Design review of the part built by this model. Coordinates are the model's own, in mm. Coordinates: 2 decimals unless noted, no trailing zeros. Write each loop counter-clockwise with the first axis right and the second up, starting at its lowest first coordinate (ties: lowest second). Pieces come first, ordered by that corner, then holes.
Q1. For probe 1 along Z at (x, y) = (-0.5, -9.25); probe 2 along Z at (x, y) = (0, -3.5); probe 3 along Y at (x, z) = (-6, 33.5), list the stretches that pass through material, from the lowest coordinate up.
Q2. Take a section at D-D (y = 1.25). Give the boundary of the cut face in (x, z), and give its area (3 significant figures).
Q3. Insertion check: pin 1 (5 mm diameter, centred on x = -1.5, y = -7, fed in from +Z); pin 2 (0.5 mm diameter, centred on y = -8.5, z = 34, fed in from -X); pin 3 (6 mm diameter, centred on x = 2.5, z = -28.5, fed in from -Y). Each pin has a flat end and moves straight along its axis. Give the tip position at first contact, or say it passes through.
Q4. Take a section at B-B (y = -5.25). Give the boundary of the cut face in (x, z), and give its area (3 significant figures).
Autodesk Fusion 360 part; units mm, degrees
sketch "Sketch1" plane through (0, 0, 0) normal (0, 1, 0) x (1, 0, 0)
  line L0 (10, 40) -> (-10, 40)
  line L1 (-10, 40) -> (-10, -40)
  line L2 (-10, -40) -> (10, -40)
  line L3 (10, -40) -> (10, 40)
  line L4 (10, 40) -> (-10, -40) construction
  line L5 (-10, 40) -> (10, -40) construction
  dimension "d1" = 20
  dimension "d2" = 80
extrude "Extrude1" add sketch "Sketch1" along normal blind 3
sketch "Sketch2" plane through (0, 0, 0) normal (0, -1, 0) x (1, 0, 0)
  line L0 (10, -40) -> (10, 40)
  line L1 (10, 40) -> (-10, 40)
  line L2 (-10, 40) -> (-10, -40)
  line L3 (-10, -40) -> (10, -40)
  line L4 (0, 48.0121) -> (0, -47.4969) construction
  line L5 (-22.9199, 34) -> (18.1137, 34) construction
  line L6 (-4.5, 35.75) -> (4.5, 35.75)
  line L7 (4.5, 35.75) -> (4.5, 34.25)
  line L8 (4.5, 34.25) -> (-4.5, 34.25)
  line L9 (-4.5, 34.25) -> (-4.5, 35.75)
  line L10 (29.4296, -34) -> (-24.7341, -34) construction
  line L11 (-4.5, -35.75) -> (4.5, -35.75)
  line L12 (4.5, -35.75) -> (4.5, -34.25)
  line L13 (4.5, -34.25) -> (-4.5, -34.25)
  line L14 (-4.5, -34.25) -> (-4.5, -35.75)
  dimension "d5" = 6
  dimension "d6" = 9
  dimension "d7" = 0.25
  dimension "d8" = 10
  dimension "d9" = 4.5
  dimension "d10" = 6
  dimension "d11" = 9
  dimension "d12" = 1.5
  dimension "d13" = 1.5
  dimension "d14" = 0.25
  dimension "d15" = 4.5
extrude "Extrude2" add sketch "Sketch2" along normal blind 10 draft -1 contours L6 L7 L8 L9 | L11 L12 L13 L14
chamfer "Chamfer1" distance 3 angle 45 4 edges at (-10, 3, 0) (0, 3, -40) (10, 3, 0) (0, 3, 40)
chamfer "Chamfer2" distance 1 angle 45 4 edges at (-4.4127, -5, -34.3373) (4.4127, -5, -34.3373) (-4.4127, -5, 34.3373) (4.4127, -5, 34.3373)
sketch "Sketch5" plane through (0, -10, 0) normal (0, -1, 0) x (1, 0, 0)
  line L0 (3.3253, 34.4246) -> (4.3254, 35.4247)
  line L1 (4.3254, 35.4247) -> (4.3254, 35.5754)
  line L2 (4.3254, 35.5754) -> (-4.3254, 35.5754)
  line L3 (-4.3254, 35.5754) -> (-4.3254, 35.4247)
  line L4 (-4.3254, 35.4247) -> (-3.3253, 34.4246)
  line L5 (-3.3253, 34.4246) -> (3.3253, 34.4246)
  line L6 (0, 34.4246) -> (1, 34.4246)
  line L7 (1, 34.4246) -> (1, 33.4246)
  line L8 (1, 33.4246) -> (0, 33.4246)
  line L9 (0, 33.4246) -> (0, 34.4246)
  line L10 (0, 34.4246) -> (-1, 34.4246)
  line L11 (-1, 34.4246) -> (-1, 33.4246)
  line L12 (-1, 33.4246) -> (0, 33.4246)
  line L13 (0, 33.4246) -> (0, 34.4246)
  dimension "d29" = 1
  dimension "d30" = 1
  dimension "d31" = 1
sketch "Sketch6" plane through (0, -10, 0) normal (0, -1, 0) x (1, 0, 0)
  line L0 (4.3254, -35.4247) -> (3.3253, -34.4246)
  line L1 (3.3253, -34.4246) -> (-3.3253, -34.4246)
  line L2 (-3.3253, -34.4246) -> (-4.3254, -35.4247)
  line L3 (-4.3254, -35.4247) -> (-4.3254, -35.5754)
  line L4 (-4.3254, -35.5754) -> (4.3254, -35.5754)
  line L5 (4.3254, -35.5754) -> (4.3254, -35.4247)
  line L6 (0, -34.4246) -> (1, -34.4246)
  line L7 (1, -34.4246) -> (1, -33.4246)
  line L8 (1, -33.4246) -> (0, -33.4246)
  line L9 (0, -33.4246) -> (0, -34.4246)
  line L10 (0, -34.4246) -> (-1, -34.4246)
  line L11 (-1, -34.4246) -> (-1, -33.4246)
  line L12 (-1, -33.4246) -> (0, -33.4246)
  line L13 (0, -33.4246) -> (0, -34.4246)
  dimension "d32" = 1
  dimension "d33" = 1
  dimension "d34" = 1
extrude "Extrude4" add sketch "Sketch5" sketch "Sketch6" against normal blind 2 contours L5 L6 L7 L8 L9 L13 | L5 L9 L10 L11 L12 L13 of sketch 2 contours L1 L6 L7 L8 L9 L13 | L1 L9 L10 L11 L12 L13
chamfer "Chamfer4" distance 0.9 angle 45 2 edges at (0, -8, -33.4246) (0, -8, 33.4246)
chamfer "Chamfer5" distance 1 angle 70 2 edges at (0, 0, 35.75) (0, 0, -35.75) measured on face at (1.1666, 0, 11.4167) measured on face at (1.1666, 0, 11.4167)
equation "d9 = d6 / 2"
equation "d15 = d11 / 2"
Response:
1. probe 1: z = -35.59 to -33.42, 33.42 to 35.59
1. probe 2: z = -35.69 to -34.31, 34.31 to 35.69
1. probe 3: y = 0 to 3
2. outline: (-8.75, -38.75) - (8.75, -38.75) - (8.75, 38.75) - (-8.75, 38.75) - close
2. area: 1,360 mm2
3. pin 1: stops at z = 35.67
3. pin 2: stops at x = -1
3. pin 3: stops at y = 0
4. outline: (-4.41, -35.66) - (4.41, -35.66) - (4.41, -35.34) - (3.41, -34.34) - (-3.41, -34.34) - (-4.41, -35.34) - close; (-4.41, 35.34) - (-3.41, 34.34) - (3.41, 34.34) - (4.41, 35.34) - (4.41, 35.66) - (-4.41, 35.66) - close
4. area: 21.2 mm2
